```python
from build123d import *

# Parameters (mm, degrees)
F0_R     = 12.5
F0_R_2   = 9.5
F1_DEPTH = 25
F2_W     = 68.8422210515
F2_H     = 15.526487492
F3_DEPTH = 25
F4_R     = 2.5
F5_DEPTH = 25
F7_W     = 5
F7_H     = 2.4230774548
F8_DEPTH = 2.5


with BuildPart() as f1:
    # F0 (on Top) → F1 (new body)
    with BuildSketch(Plane.XY):
        with BuildLine():
            Line((15.0999815878, 11.984991535), (-15.2279593776, 14.8269292644))
            Line((-15.2279593776, 14.8269292644), (-16.977902849, 14.9909110652))
            ThreePointArc((-16.977902849, 14.9909110652), (-32.4928088986, 0.4644150411), (-17.9067260562, -14.9944847833))
            Line((-17.9067260562, -14.9944847833), (-14.3728174755, -14.6704031798))
            Line((-14.3728174755, -14.6704031798), (14.7825476215, -11.9966731572))
            ThreePointArc((14.7825476215, -11.9966731572), (26.4989489041, -0.1588244182), (15.0999815878, 11.984991535))
        make_face()
        with Locations((-17.5, 0)):
            Circle(F0_R, mode=Mode.SUBTRACT)
        with Locations((14.5, 0)):
            Circle(F0_R_2, mode=Mode.SUBTRACT)
    extrude(amount=F1_DEPTH)

    # F2 (on Top) → F3 (cut)
    with BuildSketch(Plane.XY):
        with Locations((-1.8204059452, -7.763243746)):
            Rectangle(F2_W, F2_H)
    extrude(amount=F3_DEPTH, mode=Mode.SUBTRACT)

    # F4 (on face) → F5 (cut)
    with BuildSketch(Plane.XZ):
        with Locations((0, 12.5)):
            Circle(F4_R)
    extrude(amount=-F5_DEPTH, mode=Mode.SUBTRACT)

    # F7 (on offset) → F8 (cut, symmetric)
    with BuildSketch(Plane.XY.offset(12.5)):
        with Locations((0, 12.7214035019)):
            Rectangle(F7_W, F7_H)
    extrude(amount=F8_DEPTH, both=True, mode=Mode.SUBTRACT)


solid = f1.part
```
Could you check a few things on this model? Use its own coordinates, in mm. A direction names the side the tool comes from. Give positions to 0.01 mm unless a question says otherwise; leave off trailing zeros. Write each loop counter-clockwise with the first axis right and the second up, starting at its lowest first coordinate (ties: lowest second). Pieces come first, ordered by that corner, then holes. Notation, with made-up numbers: (74.25, 52.5) - (131.25, 52.5) arc R15 cw to (131.25, 77.5) - close; hole circle Ø2 at (-31.75, 50.25). An arc over 180 degrees is marked (long way). One line per item, written item: value. Start each with the question number.
Item 1: Please list where these lines run through material, in increasing order: line 1 (Z direction, x = 0, y = 5.25); line 2 (X direction, y = 5.5, z = 12.5); line 3 (X direction, y = 3.5, z = 12.5). Write a range as from..to.
Item 2: Which directions (+Z, -Z, +X, -X, +Y, -Y) give clear straight access to the entire face, cutting with the end or side of a thin tool? Please do faces 5 (the face through (1.9, 11.51, 14.5)), 6 (the face through (23.28, 8.18, 12.32)).
Item 3: Imagine slicing it at A-A, the plane y = 2.75. List the corners of the cut face in (x, z) for me, and give its area (3 significant figures).
Item 4: Imagine slicing it at B-B, the plane z = 14.25. List the corners of the cut face in (x, y) for me (3 decimals), and give its area (3 significant figures).
Item 5: If we mould it in two halves opening along Z, with no side actions, what happens to faces 1 (the face through (2.5, 12, 13)), 2 (the face through (2, 11.51, 10.5)), 3 (the face through (-0.1, 0, 9.5)), 4 (the face through (-3, 8, 0))? For each: +Z half, -Z half, draft (parallel to the pull), parting line (faces both ways), or undercut.
Item 6: Imagine slicing it at D-D, the plane z = 19. List the corners of the cut face in (x, y) for me (3 decimals).
Item 7: Imagine slicing it at C-C, the plane y = 5.75. List the corners of the cut face in (x, z) for me.
Item 8: I'm going to push flat-ended pins straight in: pin 1 (0.8 mm diameter, centred on x = 1.5, z = 10.5, fed in from +Y); pin 2 (6 mm diameter, centred on y = 10.5, z = 4, fed in from -X); pin 3 (0.8 mm diameter, centred on x = -1, z = 13.5, fed in from +Y) (3 decimals); pin 4 (12 mm diameter, centred on x = 14, z = 12, fed in from +Y). Where does each tip first touch, or does it pass through?
Geometry says:
1. line 1: 0..10, 15..25
1. line 2: -31.46..-28.72, -6.28..-2.5, 2.5..6.75, 22.25..25.17
1. line 3: -32.09..-29.5, -5.5..-2.5, 2.5..5.67, 23.33..25.98
2. face 5: +Y
2. face 6: +Z, -Z, +X, +Y
3. outline: (-32.25, 0) - (-29.69, 0) - (-29.69, 25) - (-32.25, 25) - close; (-5.31, 0) - (5.41, 0) - (5.41, 25) - (-5.31, 25) - close; (23.59, 0) - (26.18, 0) - (26.18, 25) - (23.59, 25) - close; hole circle Ø5 at (0, 12.5)
3. area: 377 mm^2
4. outline: (-32.5, 0) - (-30, 0) arc R12.5 cw to (-5, 0) - (-1.785, 0) - (-1.785, 11.51) - (-2.5, 11.51) - (-2.5, 13.634) - (-16.978, 14.991) arc R15 ccw to start; (1.785, 0) - (5, 0) arc R9.5 cw to (24, 0) - (26.5, 0) arc R12 ccw to (15.1, 11.985) - (2.5, 13.166) - (2.5, 11.51) - (1.785, 11.51) - close
4. area: 285 mm^2
5. face 1: undercut
5. face 2: undercut
5. face 3: draft
5. face 4: -Z half
6. outline: (-32.5, 0) - (-30, 0) arc R12.5 cw to (-5, 0) - (5, 0) arc R9.5 cw to (24, 0) - (26.5, 0) arc R12 ccw to (15.1, 11.985) - (-16.978, 14.991) arc R15 ccw to start
7. outline: (-31.35, 0) - (-28.6, 0) - (-28.6, 25) - (-31.35, 25) - close; (-6.4, 0) - (6.94, 0) - (6.94, 25) - (-6.4, 25) - close; (22.06, 0) - (25.03, 0) - (25.03, 25) - (22.06, 25) - close; hole circle Ø5 at (0, 12.5)
8. pin 1: y = 11.51
8. pin 2: x = -30.49
8. pin 3: through
8. pin 4: y = 12.65
